Autodesk Inventor part; units mm, degrees
ref_plane "YZ Plane" through (0, 0, 0) normal (1, 0, 0) x (0, 1, 0)
ref_plane "XZ Plane" through (0, 0, 0) normal (0, 1, 0) x (-1, 0, 0)
ref_plane "XY Plane" through (0, 0, 0) normal (0, 0, 1) x (1, 0, 0)
sketch "Sketch1" plane through (0, 0, 0) normal (0, 1, 0) x (-1, 0, 0)
  line L0 (40, 57.5) -> (-40, 57.5)
  line L1 (-40, 57.5) -> (-40, -57.5)
  line L2 (-40, -57.5) -> (40, -57.5)
  line L3 (40, -57.5) -> (40, 57.5)
  point P0 (0, 0)
  point P1 (40, 0)
  point P2 (0, 57.5)
  dimension "d0" = 115
  dimension "d1" = 80
extrude "Extrusion1" add sketch "Sketch1" along normal blind 20
sketch "Sketch12" plane through (0, 0, 0) normal (0, -1, 0) x (1, 0, 0)
  line L0 (-40, 57.5) -> (-20, 57.5)
  line L1 (-20, 57.5) -> (-20, -57.5)
  line L2 (-20, -57.5) -> (-40, -57.5)
  line L3 (-40, -57.5) -> (-40, 57.5)
  line L4 (-40, -57.5) -> (-40, 57.5)
  line L5 (0, 100.8809) -> (0, -116.5773) construction
  line L6 (40, 57.5) -> (20, 57.5)
  line L7 (20, 57.5) -> (20, -57.5)
  line L8 (20, -57.5) -> (40, -57.5)
  line L9 (40, -57.5) -> (40, 57.5)
  point P0 (0, 0)
  point P1 (-40, 0)
  point P2 (0, 0)
  point P3 (-20, 0)
  dimension "d56" = 20
  dimension "d57" = 115
extrude "Extrusion11" add sketch "Sketch12" along normal blind 37.5
sketch "Sketch13" plane through (-40, 0, 57.5) normal (-1, 0, 0) x (0, 0, 1)
  line L0 (0, 0) -> (-115, 0)
  point P0 (-57.5, 0)
  point P1 (-22.5, -15)
  point P2 (-92.5, -15)
  point P3 (-57.5, -15)
  point P4 (-57.5, 0)
  dimension "d129" = 35
  dimension "d130" = 35
  dimension "d131" = 15
hole "Hole2" at (-40, -15, 35) at (-40, -15, -35) direction (1, 0, 0) diameter 20 end through all
hole "Hole3" at (-40, -15, 0) direction (1, 0, 0) diameter 15 end through all
sketch "Sketch19" plane through (0, 20, 0) normal (0, 1, 0) x (1, 0, 0)
  point P0 (0, 0)
  point P1 (25, 0)
  point P2 (-25, 0)
  dimension "d111" = 25
  dimension "d112" = 25
hole "Hole6" at (25, 20, 0) at (-25, 20, 0) direction (0, -1, 0) diameter 15 depth 15
fillet "Fillet19" radius 20 4 edges at (-30, -37.5, -57.5) (30, -37.5, -57.5) (30, -37.5, 57.5) (-30, -37.5, 57.5)
sketch "Sketch20" plane through (0, 20, 0) normal (0, 1, 0) x (1, 0, 0)
  line L0 (-27, -22.5) -> (27, -22.5)
  line L1 (27, -22.5) -> (27, -12.5)
  line L2 (27, -12.5) -> (-27, -12.5)
  line L3 (-27, -12.5) -> (-27, -22.5)
  line L4 (-40, 57.5) -> (-40, -57.5)
  line L5 (40, -57.5) -> (40, 57.5)
  line L6 (-40, -57.5) -> (40, -57.5)
  point P0 (0, 0)
  point P1 (0, -12.5)
  dimension "d56" = 20
  dimension "d122" = 10
  dimension "d151" = 45
  dimension "d152" = 54
extrude "Extrusion15" add sketch "Sketch20" along normal blind 44
sketch "Sketch21" plane through (-40, 20, 22.5) normal (0, 0, 1) x (1, 0, 0)
  circle A0 centre (40, 22) radius 2.5
  line L0 (20, -20) -> (60, -20)
  line L1 (13, 44) -> (67, 44)
  point P0 (40, -20)
  point P1 (40, -20)
  point P2 (0, -20)
  point P3 (80, -20)
  point P4 (24.5, 37.5)
  point P5 (24.5, 6.5)
  point P6 (55.5, 6.5)
  point P7 (55.5, 37.5)
  dimension "d128" = 5
  dimension "d132" = 22
  dimension "d138" = 360
extrude "Extrusion16" cut sketch "Sketch21" against normal blind 50
sketch "Sketch24" plane through (0, 20, 0) normal (0, 1, 0) x (1, 0, 0)
  line L0 (-27, -22.5) -> (-22, -22.5)
  line L1 (-22, -22.5) -> (-22, -57.5)
  line L2 (-22, -57.5) -> (-27, -57.5)
  line L3 (-27, -57.5) -> (-27, -22.5)
  line L4 (-27, -22.5) -> (-27, -12.5)
  line L5 (27, -22.5) -> (-27, -22.5)
  line L6 (-40, -57.5) -> (40, -57.5)
  line L7 (22, -22.5) -> (27, -22.5)
  line L8 (27, -22.5) -> (27, -57.5)
  line L9 (27, -57.5) -> (22, -57.5)
  line L10 (22, -57.5) -> (22, -22.5)
  line L11 (27, -12.5) -> (27, -22.5)
  point P0 (0, 0)
  dimension "d155" = 5
  dimension "d156" = 5
extrude "Extrusion18" add sketch "Sketch24" along normal blind 44 contours L0 L1 L2 L3 | L5 L8 L6 L10
sketch "Sketch25" plane through (27, 20, 57.5) normal (1, 0, 0) x (0, 0, -1)
  line L0 (35, 44) -> (0, 0)
  line L1 (0, 44) -> (35, 44)
  line L2 (0, 44) -> (0, 0)
  line L3 (45, 0) -> (45, 44)
  point P0 (57.5, -20)
  dimension "d161" = 10
extrude "Extrusion19" cut sketch "Sketch25" against normal blind 100
properties part number "Y_Slider_Part_mit_Schrittmotor"
Can you work these out from the model? Positions are in its coordinate system, mm. A direction names the side the tool comes from. Coordinates: 2 decimals unless noted, no trailing zeros. Order: outer loops, then holes, each group sorted by start corner. A loop starts at its lowest first (then second) coordinate and runs counter-clockwise, first axis right, second up.
1. I need wall thicknesses on line 1 (X direction, y = 17, z = 0); line 2 (Z direction, x = -26.25, y = -15); line 3 (Y direction, x = 29.5, z = 35). Which ranges of each line are inside material? Lowest first, please.
2. If we section it at D-D (x = 25): Please give me the cut outline in (y, z), then the cut area to 3 significant figures.
3. If we section it at B-B (z = -35): Please give me the cut outline in (x, y), then the cut area to 3 significant figures.
4. Thinking about a two-plate mould opening in Z: for faces 6 (the face through (30, -37.5, 1)), 7 (the face through (0, 47, 12.5)), 8 (the face through (-29.9, -20.1, -5.5)), which applies, +Z half, -Z half, draft (parallel to the pull), parting line (faces both ways), or undercut?
5. If we section it at A-A (x = 0): Please give me the cut outline in (y, z), then the cut area to 3 significant figures.
6. For faces 1 (the face through (-32.436, 12.395, -0.976)), 2 (the face through (-40, -3, -1)), 3 (the face through (22, 32, 32)), 4 (the face through (27, 37, 30)), 5 (the face through (0, 0, 1)), which set-ups out of +Z, -Z, +X, -X, +Y, -Y let a thin tool reach every point of the face, with its end or its side?
7. I'm going to push flat-ended pins straight in: pin 1 (9 mm diameter, centred on x = -25, z = 0, fed in from +Y); pin 2 (22 mm diameter, centred on y = 35.5, z = 30.5, fed in from -X); pin 3 (12 mm diameter, centred on x = 28.5, z = -2, fed in from +Y); pin 4 (4 mm diameter, centred on x = 19.5, z = -1, fed in from -Y). Where does each tip first touch, or does it pass through?
8. If we section it at C-C (y = -15): Give the number of separate pieces and of enclosed holes in the cut face, then the cut area to 3 significant figures.
Entries:
1. line 1: x = -40 to -32.5, -17.5 to 17.5, 32.5 to 40
1. line 2: z = -57.5 to -45, -25 to -7.5, 7.5 to 25, 45 to 57.5
1. line 3: y = -37.5 to -25, -5 to 20
2. outline: (-37.5, -37.5) arc R20 ccw to (-17.5, -57.5) - (20, -57.5) - (20, -7.5) - (5, -7.5) - (5, 7.5) - (20, 7.5) - (20, 12.5) - (64, 12.5) - (64, 22.5) - (20, 57.5) - (-17.5, 57.5) arc R20 ccw to (-37.5, 37.5) - close; hole circle Ø20 at (-15, -35); hole circle Ø20 at (-15, 35); hole circle Ø15 at (-15, 0)
2. area: 6,620 mm2
3. outline: (-40, -37.5) - (-20, -37.5) - (-20, -25) - (-40, -25) - close; (-40, -5) - (-20, -5) - (-20, 0) - (20, 0) - (20, -5) - (40, -5) - (40, 20) - (-40, 20) - close; (20, -37.5) - (40, -37.5) - (40, -25) - (20, -25) - close
3. area: 2,300 mm2
4. face 6: draft
4. face 7: -Z half
4. face 8: undercut
5. outline: (0, -57.5) - (20, -57.5) - (20, 12.5) - (39.5, 12.5) - (39.5, 22.5) - (20, 22.5) - (20, 57.5) - (0, 57.5) - close; (44.5, 12.5) - (64, 12.5) - (64, 22.5) - (44.5, 22.5) - close
5. area: 2,690 mm2
6. face 1: +Y
6. face 2: +Z, -Z, -X, +Y, -Y
6. face 3: +Z, +Y
6. face 4: +Z, -Z, +X, +Y
6. face 5: +Z, -Z, -Y
7. pin 1: stops at y = 5
7. pin 2: stops at x = -27
7. pin 3: stops at y = 20
7. pin 4: stops at y = -37.5
8. separate pieces: 8
8. enclosed holes: 0
8. area: 2,400 mm2
